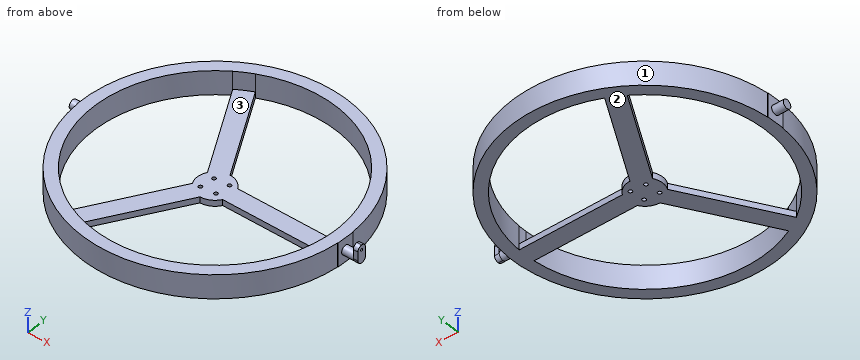
```python
from build123d import *

# Parameters (mm, degrees)
BOSS_EXTRUDE1_DEPTH = 20
SKETCH1_3_R         = 15
BOSS_EXTRUDE2_DEPTH = 5
SKETCH2_R           = 1.55
CUT_EXTRUDE1_DEPTH  = 5
SKETCH4_R           = 3.75
BOSS_EXTRUDE3_DEPTH = 10
BOSS_EXTRUDE4_START = 10
SKETCH3_R           = 3.75
BOSS_EXTRUDE4_DEPTH = 10
SKETCH5_W           = 15
SKETCH5_H           = 7.5
BOSS_EXTRUDE5_DEPTH = 4
FILLET2_R           = 3.75
SKETCH6_R           = 1
CUT_EXTRUDE2_DEPTH  = 4


with BuildPart() as part:
    # Sketch1 → Boss-Extrude1 (new body)
    with BuildSketch(Plane.XY):
        with BuildLine():
            Line((112, 7.5), (111.748601781, 7.5))
            ThreePointArc((111.748601781, 7.5), (0, 112), (-111.748601781, 7.5))
            Line((-111.748601781, 7.5), (-112, 7.5))
            Line((-112, 7.5), (-112, -7.5))
            Line((-112, -7.5), (-111.748601781, -7.5))
            ThreePointArc((-111.748601781, -7.5), (0, -112), (111.748601781, -7.5))
            Line((111.748601781, -7.5), (112, -7.5))
            Line((112, -7.5), (112, 7.5))
        make_face()
        with BuildLine():
            ThreePointArc((102, 0), (101.930949377, -3.752540346), (101.723890999, -7.5))
            ThreePointArc((101.723890999, -7.5), (51, -88.334591186), (-44.366754971, -91.845473777))
            ThreePointArc((-44.366754971, -91.845473777), (-51, -88.334591186), (-57.357136028, -84.345473777))
            ThreePointArc((-57.357136028, -84.345473777), (-102, 0), (-57.357136028, 84.345473777))
            ThreePointArc((-57.357136028, 84.345473777), (-51, 88.334591186), (-44.366754971, 91.845473777))
            ThreePointArc((-44.366754971, 91.845473777), (51, 88.334591186), (101.723890999, 7.5))
            ThreePointArc((101.723890999, 7.5), (101.930949377, 3.752540346), (102, 0))
        make_face(mode=Mode.SUBTRACT)
    extrude(amount=BOSS_EXTRUDE1_DEPTH)

    # Sketch1<3> → Boss-Extrude2 (add)
    with BuildSketch(Plane.XY):
        with BuildLine():
            Line((-57.357136028, 84.345473777), (-12.990381057, 7.5))
            ThreePointArc((-12.990381057, 7.5), (-7.5, 12.990381057), (0, 15))
            Line((0, 15), (-44.366754971, 91.845473777))
            ThreePointArc((-44.366754971, 91.845473777), (-51, 88.334591186), (-57.357136028, 84.345473777))
        make_face()
        Circle(SKETCH1_3_R)
        with BuildLine():
            Line((-44.366754971, -91.845473777), (0, -15))
            ThreePointArc((0, -15), (-7.5, -12.990381057), (-12.990381057, -7.5))
            Line((-12.990381057, -7.5), (-57.357136028, -84.345473777))
            ThreePointArc((-57.357136028, -84.345473777), (-51, -88.334591186), (-44.366754971, -91.845473777))
        make_face()
        with BuildLine():
            ThreePointArc((15, 0), (14.488887394, -3.882285677), (12.990381057, -7.5))
            Line((12.990381057, -7.5), (101.723890999, -7.5))
            ThreePointArc((101.723890999, -7.5), (101.930949377, -3.752540346), (102, 0))
            ThreePointArc((102, 0), (101.930949377, 3.752540346), (101.723890999, 7.5))
            Line((101.723890999, 7.5), (12.990381057, 7.5))
            ThreePointArc((12.990381057, 7.5), (14.488887394, 3.882285677), (15, 0))
        make_face()
    extrude(amount=BOSS_EXTRUDE2_DEPTH)

    # Sketch2 → Cut-Extrude1 (cut)
    with BuildSketch(Plane.XY.offset(5)):
        with Locations((-5.656854249, 5.656854249)):
            Circle(SKETCH2_R)
        with Locations((6.717514421, 6.717514421)):
            Circle(SKETCH2_R)
        with Locations((5.656854249, -5.656854249)):
            Circle(SKETCH2_R)
        with Locations((-6.717514421, -6.717514421)):
            Circle(SKETCH2_R)
    extrude(amount=-CUT_EXTRUDE1_DEPTH, mode=Mode.SUBTRACT)

    # Sketch4 → Boss-Extrude3 (add)
    with BuildSketch(Plane.ZY.offset(112)):
        with Locations(Location((10, 0, 0), (0, 0, 180))):
            Circle(SKETCH4_R)
    extrude(amount=BOSS_EXTRUDE3_DEPTH)

    # Sketch3 → Boss-Extrude4 (add)
    with BuildSketch(Plane(origin=(112, 0, 0), x_dir=(0, 0, -1), z_dir=(1, 0, 0)).offset(BOSS_EXTRUDE4_START)):
        with Locations((-10, 0)):
            Circle(SKETCH3_R)
    extrude(amount=-BOSS_EXTRUDE4_DEPTH)

    # Sketch5 → Boss-Extrude5 (add)
    with BuildSketch(Plane(origin=(122, 0, 0), x_dir=(0, 0, -1), z_dir=(1, 0, 0))):
        with Locations((-13.75, 0)):
            Rectangle(SKETCH5_W, SKETCH5_H)
    extrude(amount=BOSS_EXTRUDE5_DEPTH)

    # Fillet2
    fillet2_edges = [part.edges().sort_by_distance(p)[0] for p in [
        (124, -3.75, 21.25),
        (124, 3.75, 21.25),
        (124, 3.75, 6.25),
        (124, -3.75, 6.25),
    ]]
    fillet(fillet2_edges, radius=FILLET2_R - 0.0001)  # a hair under: the kernel refuses the full size

    # Sketch6 → Cut-Extrude2 (cut)
    with BuildSketch(Plane(origin=(126, 0, 0), x_dir=(0, 0, -1), z_dir=(1, 0, 0))):
        with Locations((-17.25, 0)):
            Circle(SKETCH6_R)
    extrude(amount=-CUT_EXTRUDE2_DEPTH, mode=Mode.SUBTRACT)


solid = part.part
```
Geometry check sheet. Reference: the model listing, model coordinates, mm. Face numbers are marked on the shaded views. Coordinates: 2 decimals unless noted, no trailing zeros. Order: outer loops, then holes, each group sorted by start corner. A loop starts at its lowest first (then second) coordinate and runs counter-clockwise, first axis right, second up. Notation, with made-up numbers: (72, -16.5) - (84, -16.5) arc R34 cw to (84, 16.5) - close; hole circle Ø8 at (8, 43.25). An arc over 180 degrees is marked (long way). Answer as a JSON object with one key per item and string values. Group by question number.
Item 1: Sectioned sample at C-C, the plane x = 59.5. Record the cut outline in (y, z).
Item 2: Sectioned sample at D-D, the plane y = 95. Record the cut outline in (x, z), and give its area (3 significant figures).
Item 3: Sectioned sample at A-A, the plane y = 27.5. Record the cut outline in (x, z), and give its area (3 significant figures).
Item 4: Draft check along X on the marked faces 1, 2 and 3. Enter one of: +X half, -X half, draft (parallel to the pull), parting line (faces both ways), or undercut.
Item 5: Depth check by flat-ended pin: pin 1 Ø3 at (x, z) = (-40, 2.5) entering from -Y; pin 2 Ø3 at (x, z) = (27, 10.5) entering from +Y; pin 3 Ø1.6 at (y, z) = (0, 17.25) entering from -X; pin 4 Ø1.9 at (x, y) = (-5.66, 5.66) entering from +Z. Enter the tip coordinate at first touch or a pass-through.
Item 6: Sectioned sample at B-B, the plane x = -72.5. Record the cut outline in (y, z), and give its area (3 significant figures).
Item 7: Scan lines: probe 1 along Y at (x, z) = (85, 13); probe 2 along Z at (x, y) = (-19, -24); probe 3 along Z at (x, y) = (110, 15). Record each from-to range of solid material in increasing order.
Resolved:
{
 "1": {"outline": "(-94.89, 0) - (-82.85, 0) - (-82.85, 20) - (-94.89, 20) - close; (-7.5, 0) - (7.5, 0) - (7.5, 5) - (-7.5, 5) - close; (82.85, 0) - (94.89, 0) - (94.89, 20) - (82.85, 20) - close"},
 "2": {"outline": "(-59.32, 0) - (-37.13, 0) - (-37.13, 20) - (-59.32, 20) - close; (37.13, 0) - (59.32, 0) - (59.32, 20) - (37.13, 20) - close", "area": "887 mm^2"},
 "3": {"outline": "(-108.57, 0) - (-98.22, 0) - (-98.22, 20) - (-108.57, 20) - close; (-24.54, 0) - (-7.22, 0) - (-7.22, 5) - (-24.54, 5) - close; (98.22, 0) - (108.57, 0) - (108.57, 20) - (98.22, 20) - close", "area": "501 mm^2"},
 "4": {"face 1": "parting line", "face 2": "draft", "face 3": "undercut"},
 "5": {"pin 1": "y = -105.17", "pin 2": "y = 109.06", "pin 3": "x = -112", "pin 4": "through"},
 "6": {"outline": "(-85.37, 0) - (-71.75, 0) - (-71.75, 20) - (-85.37, 20) - close; (71.75, 0) - (85.37, 0) - (85.37, 20) - (71.75, 20) - close", "area": "545 mm^2"},
 "7": {"probe 1": "-72.93 to -56.38, 56.38 to 72.93", "probe 2": "0 to 5", "probe 3": "0 to 20"}
}
